Here's how the part is built. I have some questions about the finished solid (model axes, mm). A direction names the side the tool comes from. Round coordinates to 2 decimals unless told otherwise and drop trailing zeros. Order: outer loops, then holes, each group sorted by start corner. A loop starts at its lowest first (then second) coordinate and runs counter-clockwise, first axis right, second up. Notation, with made-up numbers: (31.5, 10) -> (55.5, 10) arc R20 cw to (55.5, 30) -> close; hole circle Ø11 at (62, 60.5). An arc over 180 degrees is marked (long way). Use a Markdown table: item, result. Add a question column.
(1) If I drill on probe 1 along Y at (x, z) = (15, 1); probe 2 along X at (y, z) = (-4.5, 3.75); probe 3 along X at (y, z) = (-3, 6.75), over which ranges is the centre line in solid material (lowest first)?
(2) Thinking about a two-plate mould opening in X: for faces 1 (the face through (-13, -2, -4.5)), 2 (the face through (-13, -2, 3)), 3 (the face through (-21.797, -0.07, 6.859)), which applies, pulls with the +X half, pulls with the -X half, needs draft (parallel to the pull), parting line crosses it, or undercut?
(3) I want a section at C-C, the plane x = -15. Please give me the cut outline in (y, z).
(4) I want a section at D-D, the plane x = -0.5. Please give me the cut outline in (y, z).
(5) On a 3-axis mill with a long thin cutter (end or side, diameter ignored), from which of +Z, -Z, +X, -X, +Y, -Y can I reach the whole of each face in a straight line? I mean faces 4 (the face through (11.254, 0.165, -2.218)), 5 (the face through (0, 0, 4)), 6 (the face through (0, 0, 8)), 7 (the face through (-19, 0, 6)). Say none if no direction works.
(6) I want a section at A-A, the plane y = 0. Give the number of separate pieces and of enclosed holes in the cut face, then the cut area to 3 significant figures.
(7) I want a section at B-B, the plane z = 1.5. Please give me the cut outline in (x, y).
(8) I'm going to push flat-ended pins straight in: P1, Ø1.5, axis at x = -16.5, y = -2, coming from the +Z side; P2, Ø2, axis at y = 2, z = -1.5, coming from the +X side. Where does each tip first touch, or does it pass through?
Autodesk Inventor part; units mm, degrees
ref_plane "YZ Plane" through (0, 0, 0) normal (1, 0, 0) x (0, 1, 0)
ref_plane "XZ Plane" through (0, 0, 0) normal (0, 1, 0) x (-1, 0, 0)
ref_plane "XY Plane" through (0, 0, 0) normal (0, 0, 1) x (1, 0, 0)
sketch "Szkic1" plane through (0, 0, 0) normal (0, 0, 1) x (1, 0, 0)
  line L0 (-23, -5) -> (23, -5)
  line L1 (23, -5) -> (23, 5)
  line L2 (23, 5) -> (-23, 5)
  line L3 (-23, 5) -> (-23, -5)
  line L4 (-23, -5) -> (23, 5) construction
  line L5 (23, -5) -> (-23, 5) construction
  circle A0 centre (-15, 0) radius 3.75
  circle A1 centre (-15, 0) radius 2.25
  circle A2 centre (15, 0) radius 3.75
  circle A3 centre (15, 0) radius 2.25
  line L6 (-6, -5) -> (6, -5)
  line L7 (6, -5) -> (6, 5)
  line L8 (6, 5) -> (-6, 5)
  line L9 (-6, 5) -> (-6, -5)
  line L10 (-6, -5) -> (6, 5) construction
  line L11 (6, -5) -> (-6, 5) construction
  circle A4 centre (-15, 0) radius 4
  circle A5 centre (15, 0) radius 4
  point P0 (0, 0)
  point P1 (0, 0)
  dimension "d1" = 10
  dimension "d3" = 7.5
  dimension "d4" = 4.5
  dimension "d6" = 15
  dimension "d7" = 15
  dimension "d8" = 8
  dimension "d9" = 6
  dimension "d18" = 8
  dimension "d19" = 8
extrude "Wyciągnięcie proste1" add sketch "Szkic1" along normal blind 8 contours L3 L2 L9 L0 | L9 L2 L7 L0 | L7 L2 L1 L0 | A0 | A1 | A2 | A3 | A4 | A5
extrude "Wyciągnięcie proste2" cut sketch "Szkic1" along normal blind 4 contours L9 L2 L7 L0
extrude "Wyciągnięcie proste3" cut sketch "Szkic1" along normal through all contours A1 | A3
extrude "Wyciągnięcie proste4" add sketch "Szkic1" against normal blind 4.5 contours A0 | A2
extrude "Wyciągnięcie proste5" cut sketch "Szkic1" against normal blind 5 from surface at 8 contours A0 | A1 | A2 | A3 | A4 | A5
fillet "Zaokrąglenie1" radius 4 2 edges at (23, 0, 8) (-23, 0, 8)
properties part number "ZTopCable" material "Tworzywo sztuczne ABS"
Taken from the geometry:
| question | item | result |
|---|---|---|
| 1 | probe 1 | y = -5 to -2.25, 2.25 to 5 |
| 1 | probe 2 | x = -23 to -6, 6 to 23 |
| 1 | probe 3 | x = -21.91 to -17.65, -12.35 to 12.35, 17.65 to 21.91 |
| 2 | face 1 | needs draft |
| 2 | face 2 | undercut |
| 2 | face 3 | pulls with the -X half |
| 3 | outline | (-5, 0) -> (-3.75, 0) -> (-3.75, -4.5) -> (-2.25, -4.5) -> (-2.25, 3) -> (-4, 3) -> (-4, 8) -> (-5, 8) -> close; (2.25, -4.5) -> (3.75, -4.5) -> (3.75, 0) -> (5, 0) -> (5, 8) -> (4, 8) -> (4, 3) -> (2.25, 3) -> close |
| 4 | outline | (-5, 4) -> (5, 4) -> (5, 8) -> (-5, 8) -> close |
| 5 | face 4 | -Z |
| 5 | face 5 | -Z, +Y, -Y |
| 5 | face 6 | +Z, +X, -X, +Y, -Y |
| 5 | face 7 | +Z |
| 6 | separate pieces | 3 |
| 6 | enclosed holes | 0 |
| 6 | area | 233 mm2 |
| 7 | outline | (-23, -5) -> (-6, -5) -> (-6, 5) -> (-23, 5) -> close; (6, -5) -> (23, -5) -> (23, 5) -> (6, 5) -> close; hole circle Ø4.5 at (-15, 0); hole circle Ø4.5 at (15, 0) |
| 8 | P1 | stops at z = 3 |
| 8 | P2 | stops at x = 18.61 |
